For this review, take the finished solid that the model builds, in its own axes (mm). Coordinates: 2 decimals unless noted, no trailing zeros. Write each loop counter-clockwise with the first axis right and the second up, starting at its lowest first coordinate (ties: lowest second). Pieces come first, ordered by that corner, then holes. Notation, with made-up numbers: (85.25, 60.25) -> (118.25, 60.25) arc R33 ccw to (118.25, 90.25) -> close; hole circle Ø8 at (69, 73). An arc over 180 degrees is marked (long way). One line per item, written item: value. Start each with the question number.
1) Add section C-C (z = 0.3). State the section outline as (x, y) points, and give its area (3 significant figures).
2) For probe 1 along Y at (x, z) = (0, 0.9); probe 2 along X at (y, z) = (0.4, 0.1); probe 3 along Y at (x, z) = (0.85, 1.25), list the stretches that pass through material, from the lowest coordinate up. Write a range as from..to.
3) For pin 1 Ø3 at (x, y) = (0, 0) entering from -Z, flat-tipped, find the tip position at first contact; note if it passes through.
4) Mouldability with a two-part tool opening along X and no side actions: class faces 1 (the flat face through (-1, -1, 0)), 2 (the cylindrical face through (-0.748, 0.976, 1.191)) as released by +X, released by -X, zero draft, split by the parting line, or undercut.
5) Add section A-A (x = 0). State the section outline as (y, z) points.
6) Add section B-B (z = 0.9). State the section outline as (x, y) points.
Solid Edge part; units mm, degrees
sketch "Sketch1" plane through (0, 0, 0) normal (0, 0, 1) x (1, 0, 0)
  line L0 (-1.5, -2.5981) -> (0, -2.5981)
  line L1 (1.5, -2.5981) -> (0, -2.5981)
  line L2 (1.5, -2.5981) -> (2.25, -1.299)
  line L3 (3, 0) -> (2.25, -1.299)
  line L4 (3, 0) -> (2.25, 1.299)
  line L5 (1.5, 2.5981) -> (2.25, 1.299)
  line L6 (1.5, 2.5981) -> (0, 2.5981)
  line L7 (-1.5, 2.5981) -> (0, 2.5981)
  line L8 (-1.5, 2.5981) -> (-2.25, 1.299)
  line L9 (-3, 0) -> (-2.25, 1.299)
  line L10 (-3, 0) -> (-2.25, -1.299)
  line L11 (-1.5, -2.5981) -> (-2.25, -1.299)
extrude "Protrusion1" add sketch "Sketch1" along normal blind 2.35
sketch "Sketch2" plane through (0, 0, 0) normal (1, 0, 0) x (0, 1, 0)
  line L0 (2.2294, 2.5739) -> (3.6283, 1.175)
  line L1 (2.2294, -0.2239) -> (3.6283, 1.175)
revolve "RevolvedCutout1" cut sketch "Sketch2" angle 360 about axis through (0, 0, -57) along (0, 0, 1) material side at (0, 2.9642, 1.9098)
hole "Hole_1" at (0, 0, 2.35) direction (0, 0, -1) diameter 2.459 end up to next thread major 3 thread length 2
properties material "Stainless steel"
Numbers:
1. outline: (-2.71, -0.51) -> (-2.25, -1.3) -> (-1.79, -2.09) arc R2.75 ccw to (-0.91, -2.6) -> (0.91, -2.6) arc R2.75 ccw to (1.79, -2.09) -> (2.25, -1.3) -> (2.71, -0.51) arc R2.75 ccw to (2.71, 0.51) -> (2.25, 1.3) -> (1.79, 2.09) arc R2.75 ccw to (0.91, 2.6) -> (-0.91, 2.6) arc R2.75 ccw to (-1.79, 2.09) -> (-2.25, 1.3) -> (-2.71, 0.51) arc R2.75 ccw to start; hole circle Ø2.46 at (0, 0)
1. area: 17.9 mm²
2. probe 1: -2.6..-1.23, 1.23..2.6
2. probe 2: -2.52..-1.16, 1.16..2.52
2. probe 3: -2.6..-0.89, 0.89..2.6
3. pin 1: z = 0
4. face 1: zero draft
4. face 2: undercut
5. outline: (-2.6, 0.14) -> (-2.45, 0) -> (-1.23, 0) -> (-1.23, 2.35) -> (-2.45, 2.35) -> (-2.6, 2.21) -> close; (1.23, 0) -> (2.45, 0) -> (2.6, 0.14) -> (2.6, 2.21) -> (2.45, 2.35) -> (1.23, 2.35) -> close
6. outline: (-3, 0) -> (-2.25, -1.3) -> (-1.5, -2.6) -> (1.5, -2.6) -> (2.25, -1.3) -> (3, 0) -> (2.25, 1.3) -> (1.5, 2.6) -> (-1.5, 2.6) -> (-2.25, 1.3) -> close; hole circle Ø2.46 at (0, 0)
